Part print with two shaded views. Sizes in mm from the minimum x, y, z corner. Round coordinates to 2 decimals unless told otherwise and drop trailing zeros. Order: outer loops, then holes, each group sorted by start corner. A loop starts at its lowest first (then second) coordinate and runs counter-clockwise, first axis right, second up. Notation, with made-up numbers: M -28,-30.5 L 19,-30.5 A23 cw 19,5.5 Z; hole C 17,40 d10. An arc over 180 degrees is marked long. Return JSON: item names as keys, results as strings. Group by question number.
Item 1: Slice it at B-B on x = 75. Write the cut outline in (y, z), then the cut area to 3 significant figures.
Item 2: Slice it at A-A on y = 5. Write the cut outline in (x, z), then the cut area to 3 significant figures.
Item 3: Probe line 1 along X through (y, z) = (5, 13); line 2 along Y through (x, z) = (5, 30). List the from-to ranges inside material, lowest first.
Item 4: Pin check, flat tips, straight feed: pin 1 Ø3.5 at (x, y) = (75, 5) entering from +Z; pin 2 Ø4 at (x, y) = (10, 86) entering from -Z. Stop position of each tip, or through.
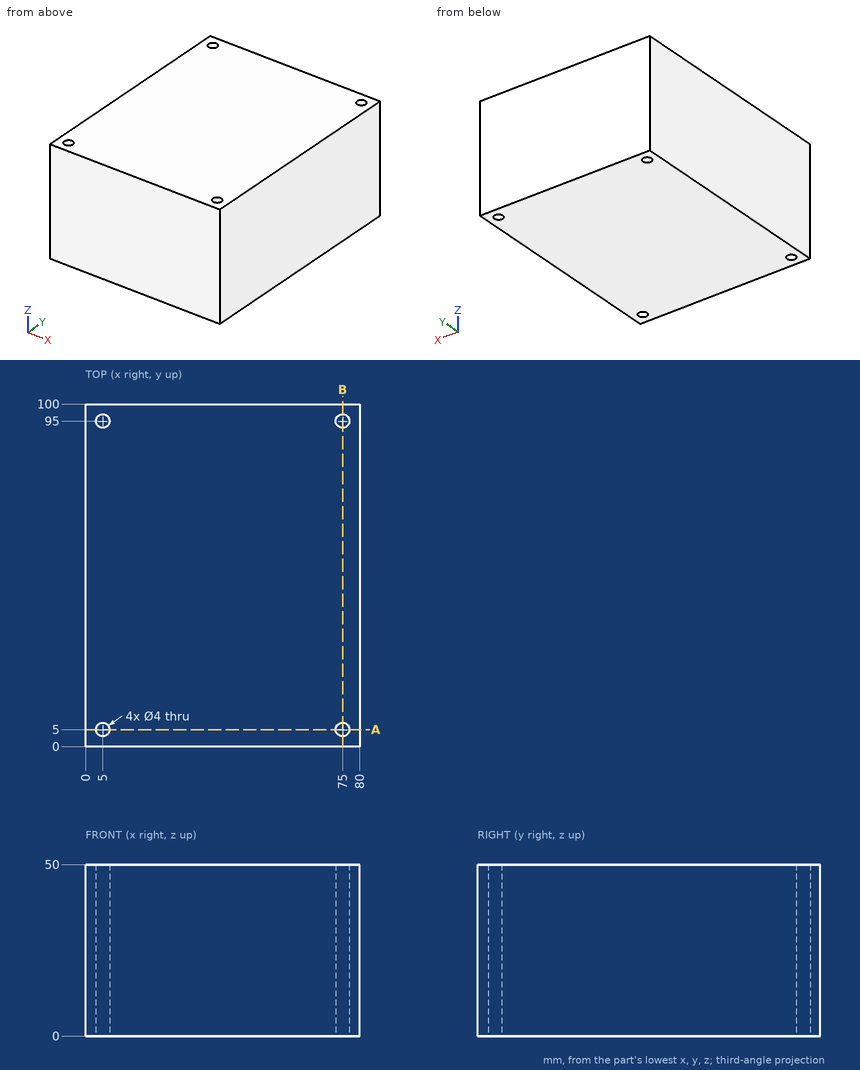
Output values:
{
 "1": {"outline": "M 0,0 L 3,0 L 3,50 L 0,50 Z; M 7,0 L 93,0 L 93,50 L 7,50 Z; M 97,0 L 100,0 L 100,50 L 97,50 Z", "area": "4,600 mm²"},
 "2": {"outline": "M 0,0 L 3,0 L 3,50 L 0,50 Z; M 7,0 L 73,0 L 73,50 L 7,50 Z; M 77,0 L 80,0 L 80,50 L 77,50 Z", "area": "3,600 mm²"},
 "3": {"line 1": "0 to 3, 7 to 73, 77 to 80", "line 2": "0 to 3, 7 to 93, 97 to 100"},
 "4": {"pin 1": "through", "pin 2": "z = 0"}
}
